Geometry check sheet. Reference: the model listing, model coordinates, mm. Give positions to 0.01 mm unless a question says otherwise; leave off trailing zeros. Order: outer loops, then holes, each group sorted by start corner. A loop starts at its lowest first (then second) coordinate and runs counter-clockwise, first axis right, second up. Notation, with made-up numbers: M 85.25,-1.75 L 128.25,-1.75 A19 cw 128.25,27.25 Z; hole C 19,21 d5. An arc over 180 degrees is marked long. Put each result on its own line as item: value. Start each with the question number.
Q1. Section check B-B on x = 43.5. Record the cut outline in (y, z).
Q2. Material ranges on L1, parallel to Z at x = -132.5, y = -2; L2, parallel to Z at x = -425.5, y = -2.5; L3, parallel to Z at x = 201, y = -1.5, recorded low to high.
Q3. Section check A-A on z = -9. Record the cut outline in (x, y).
Q4. Go/stop test with a flat-tipped pin: pin 1 (7 mm diameter, centred on x = -132.5, z = -245, fed in from +Y). Record where the tip stops, or that it passes through.
Q5. Section check C-C on y = 2.75. State how many separate pieces and enclosed holes the cut face has, then the cut area to 3 significant figures.
```python
from build123d import *

# Parameters (mm, degrees)
SKETCH1_W               = 960
SKETCH1_H               = 510
BOSS_EXTRUDE1_DEPTH     = 7.5
SKETCH3_W               = 580
SKETCH3_H               = 250
CUT_EXTRUDE1_DEPTH      = 16
ESQUISSE3_R             = 4.5
ENL_V_MAT_EXTRU_2_DEPTH = 16


with BuildPart() as part:
    # Sketch1 → Boss-Extrude1 (new body, symmetric)
    with BuildSketch(Plane(origin=(0, 0, 0), x_dir=(1, 0, 0), z_dir=(0, 1, 0))):
        Rectangle(SKETCH1_W, SKETCH1_H)
    extrude(amount=BOSS_EXTRUDE1_DEPTH, both=True)

    # Sketch3 → Cut-Extrude1 (cut, through all)
    with BuildSketch(Plane(origin=(0, 7.5, 0), x_dir=(1, 0, 0), z_dir=(0, 1, 0))):
        with Locations((164.54751, 120)):
            Rectangle(SKETCH3_W, SKETCH3_H)
    extrude(amount=-CUT_EXTRUDE1_DEPTH, mode=Mode.SUBTRACT)

    # Esquisse3 → Enlèv. mat.-Extru.2 (cut, through all)
    with BuildSketch(Plane.XZ.offset(7.5)):
        with Locations((-425.5, 228)):
            Circle(ESQUISSE3_R)
        with Locations((-425.5, 128)):
            Circle(ESQUISSE3_R)
        with Locations((-325.5, 128)):
            Circle(ESQUISSE3_R)
        with Locations((-325.5, 228)):
            Circle(ESQUISSE3_R)
        with Locations((-132.5, 10)):
            Circle(ESQUISSE3_R)
        with Locations((-132.5, -245)):
            Circle(ESQUISSE3_R)
        with Locations((467.5, -245)):
            Circle(ESQUISSE3_R)
        with Locations((467.5, 10)):
            Circle(ESQUISSE3_R)
    extrude(amount=-ENL_V_MAT_EXTRU_2_DEPTH, mode=Mode.SUBTRACT)


solid = part.part
```
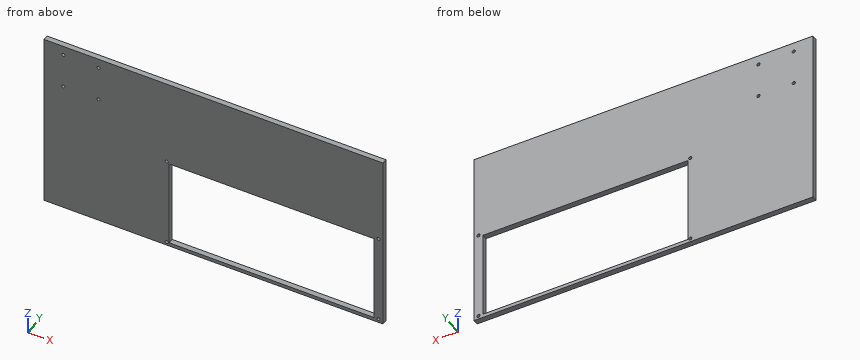
Results found:
1. outline: M -7.5,-255 L 7.5,-255 L 7.5,-245 L -7.5,-245 Z; M -7.5,5 L 7.5,5 L 7.5,255 L -7.5,255 Z
2. L1: z = -255 to -249.5, -240.5 to 5.5, 14.5 to 255
2. L2: z = -255 to 123.5, 132.5 to 223.5, 232.5 to 255
2. L3: z = -255 to -245, 5 to 255
3. outline: M -480,-7.5 L -125.45,-7.5 L -125.45,7.5 L -480,7.5 Z; M 454.55,-7.5 L 480,-7.5 L 480,7.5 L 454.55,7.5 Z
4. pin 1: passes through
5. separate pieces: 1
5. enclosed holes: 9
5. area: 344,000 mm^2
